Study the drawing (mm; zero at the part's minimum x, y, z) and answer. Coordinates: 2 decimals unless noted, no trailing zeros. Loops run counter-clockwise (first coordinate to the right, second up) from the corner with the lowest first, then second, coordinate; pieces in that order, holes last. Notation, with made-up numbers: (-11, 80.25) -> (19, 80.25) arc R13 ccw to (19, 101.25) -> close; hole circle Ø3 at (7, 54). An arc over 180 degrees is marked (long way). Answer as CSV lines item,"result".
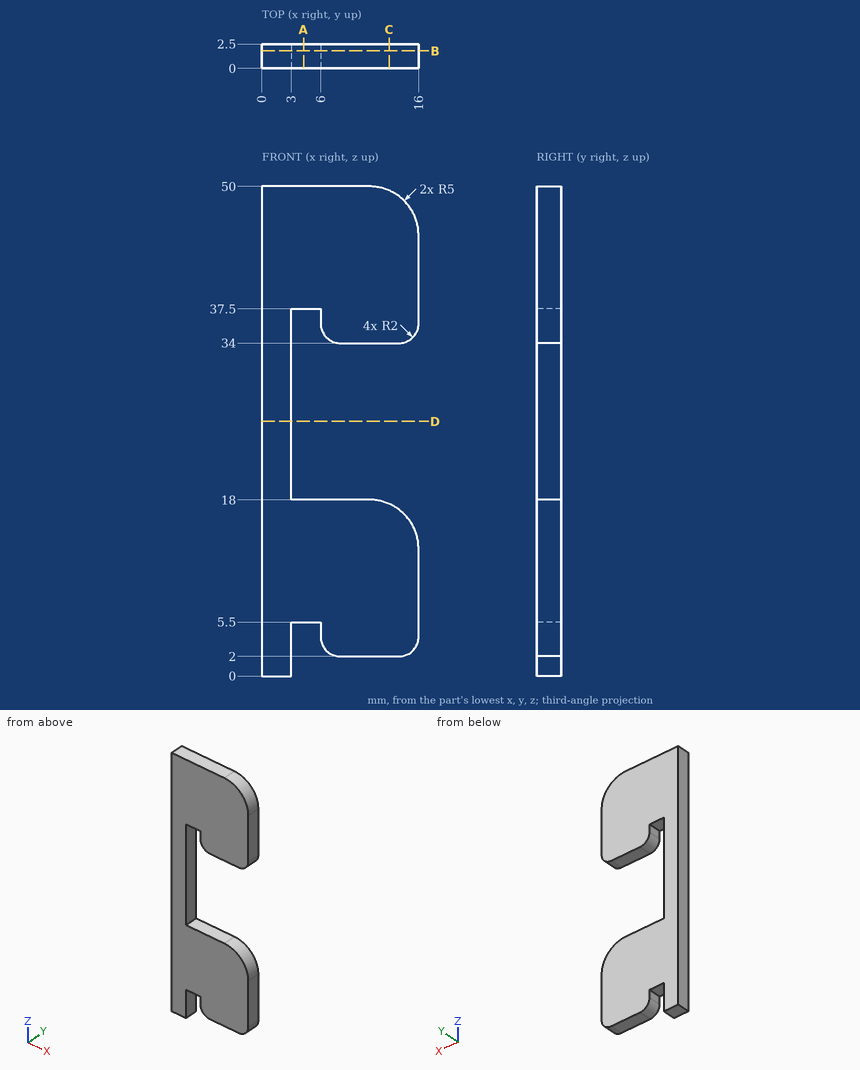
Q1. A cutting plane is placed at C-C, the plane x = 13. Write down the section's boundary in (y, z), and give its area (3 significant figures).
Results:
outline,"(0, 2) -> (2.5, 2) -> (2.5, 17.58) -> (0, 17.58) -> close; (0, 34) -> (2.5, 34) -> (2.5, 49.58) -> (0, 49.58) -> close"
area,"77.9 mm²"
Q2. Find the intervals of material crossed by probe 1 along Z at (x, y) = (8.75, 0.55); probe 2 along X at (y, z) = (2.4, 36.5); probe 3 along Z at (x, y) = (14, 2.25), in increasing order. Write a range as [from, to].
Results:
probe 1,"z = [2, 18], [34, 50]"
probe 2,"x = [0, 3], [6, 16]"
probe 3,"z = [2, 17], [34, 49]"
Q3. Given pin 1 Ø0.8 at (x, y) = (5, 1) entering from -Z; pin 2 Ø0.8 at (y, z) = (1, 28.5) entering from +X; pin 3 Ø0.8 at (y, z) = (2, 3.5) entering from +X, each flat-ended and moving along its own axis, determine where each tip first touches the part or whether it passes through.
Results:
pin 1,"stops at z = 5.5"
pin 2,"stops at x = 3"
pin 3,"stops at x = 16"
Q4. A cutting plane is placed at D-D, the plane z = 26. Write down the section's boundary in (x, y), and give its area (3 significant figures).
Results:
outline,"(0, 0) -> (3, 0) -> (3, 2.5) -> (0, 2.5) -> close"
area,"7.50 mm²"
Q5. A cutting plane is placed at A-A, the plane x = 4.25. Write down the section's boundary in (y, z).
Results:
outline,"(0, 5.5) -> (2.5, 5.5) -> (2.5, 18) -> (0, 18) -> close; (0, 37.5) -> (2.5, 37.5) -> (2.5, 50) -> (0, 50) -> close"
Q6. A cutting plane is placed at B-B, the plane y = 1.8. Write down the section's boundary in (x, z).
Results:
outline,"(0, 0) -> (3, 0) -> (3, 5.5) -> (6, 5.5) -> (6, 4) arc R2 ccw to (8, 2) -> (14, 2) arc R2 ccw to (16, 4) -> (16, 13) arc R5 ccw to (11, 18) -> (3, 18) -> (3, 37.5) -> (6, 37.5) -> (6, 36) arc R2 ccw to (8, 34) -> (14, 34) arc R2 ccw to (16, 36) -> (16, 45) arc R5 ccw to (11, 50) -> (0, 50) -> close"
